Geometry: final body of the model. Coordinates: model frame, mm. A direction names the side the tool comes from. Round coordinates to 2 decimals unless told otherwise and drop trailing zeros. Loops run counter-clockwise (first coordinate to the right, second up) from the corner with the lowest first, then second, coordinate; pieces in that order, holes last. Notation, with made-up numbers: (-3, -24.5) - (3, -24.5) arc R32 cw to (3, 13.5) - close; hole circle Ø2 at (78.25, -4.75). An arc over 180 degrees is marked (long way). Answer as a JSON object with one key per item and string values. Group by question number.
Item 1: Line query: line 1 (Y direction, x = -15, z = -4.5); line 2 (X direction, y = 0.5, z = 7.75); line 3 (Y direction, x = -96, z = 1). Output: solid intervals per line, ascending.
Item 2: First-contact query: pin 1 (10 mm diameter, centred on x = -30, y = -24, fed in from -Z); pin 2 (8 mm diameter, centred on x = -88, y = 7.5, fed in from +Z); pin 3 (5 mm diameter, centred on x = -97, y = 13.5, fed in from +Z); pin 4 (3 mm diameter, centred on y = 6.5, z = -5.5, fed in from +X). Flat tips, straight axial feed; report the tip coordinate or a pass-through.
Item 3: Reachability of faces 1 (the face through (-9, -1, -0.042)), 2 (the face through (-102, 0, 5)), 3 (the face through (-82, 19, -4)), 4 (the face through (-3, 11, 6.958)) from +Z, -Z, +X, -X, +Y, -Y: full face, straight path, thin tool, end or side. Return the list, or none.
Item 4: Draft query along X for faces 5 (the face through (-102, 20, 5)), 6 (the face through (-82, -21, -4)), 7 (the face through (-2.292, 10.2, 7.4)), 8 (the face through (-72.292, -1, -4)). Return one class per face: released by +X, released by -X, zero draft, split by the parting line, or undercut.
Item 5: Section B-B (x = -33.5). Return the cut outline in (y, z).
Item 6: Section A-A (y = -22.5). Return the cut outline in (x, z).
```python
from build123d import *

# Parameters (mm, degrees)
BOSS_EXTRUDE1_DEPTH = 20
FILLET1_R           = 1
SKETCH2_R           = 9
CUT_EXTRUDE1_DEPTH  = 20
BOSS_EXTRUDE2_START = 2
BOSS_EXTRUDE2_DEPTH = 2
SKETCH4_W           = 20
SKETCH4_H           = 20
BOSS_EXTRUDE3_DEPTH = 2
FILLET2_R           = 1
SKETCH5_W           = 12.5
SKETCH5_H           = 2
CUT_EXTRUDE2_DEPTH  = 24
BOSS_EXTRUDE4_DEPTH = 80
FILLET3_R           = 1
SKETCH8_R           = 7.11392485
SKETCH8_W           = 20
SKETCH8_H           = 40
CUT_EXTRUDE3_DEPTH  = 2
SKETCH9_W           = 20
SKETCH9_H           = 2
BOSS_EXTRUDE5_DEPTH = 16
FILLET4_R           = 1
SKETCH10_R          = 2.5
CUT_EXTRUDE4_DEPTH  = 20


with BuildPart() as part:
    # Sketch1 → Boss-Extrude1 (new body)
    with BuildSketch(Plane(origin=(0, 0, 0), x_dir=(1, 0, 0), z_dir=(0, 1, 0))):
        Polygon((-2.291666667, 11.041666667), (-22.291666667, 11.041666667), (-22.291666667, -8.958333333), (-2.291666667, -8.958333333), (-2.291666667, -6.958333333), (-20.291666667, -6.958333333), (-20.291666667, 9.041666667), (-2.291666667, 9.041666667), align=None)
    extrude(amount=BOSS_EXTRUDE1_DEPTH)

    # Fillet1
    fillet1_edges = [part.edges().sort_by_distance(p)[0] for p in [
        (-22.291666667, 10, 8.958333333),
        (-22.291666667, 10, -11.041666667),
    ]]
    fillet(fillet1_edges, radius=FILLET1_R)

    # Sketch2 → Cut-Extrude1 (cut)
    with BuildSketch(Plane.XY.offset(8.958333333)):
        with Locations(Location((-12.291666667, 10, 0), (0, 0, 180))):
            Circle(SKETCH2_R)
    extrude(amount=-CUT_EXTRUDE1_DEPTH, mode=Mode.SUBTRACT)

    # Sketch3 → Boss-Extrude2 (add)
    with BuildSketch(Plane(origin=(0, 20, 0), x_dir=(1, 0, 0), z_dir=(0, 1, 0)).offset(BOSS_EXTRUDE2_START)):
        Polygon((-2.291666667, 2.377848536), (-2.291666667, 9.041666667), (-20.291666667, 9.041666667), (-20.291666667, -6.958333333), (-2.291666667, -6.958333333), (-2.291666667, 0.377848536), align=None)
        with BuildLine():
            Line((-2.291666667, 9.041666667), (-2.291666667, 11.041666667))
            Line((-2.291666667, 11.041666667), (-21.291666667, 11.041666667))
            ThreePointArc((-21.291666667, 11.041666667), (-21.998773448, 10.748773448), (-22.291666667, 10.041666667))
            Line((-22.291666667, 10.041666667), (-22.291666667, -7.958333333))
            ThreePointArc((-22.291666667, -7.958333333), (-21.998773448, -8.665440115), (-21.291666667, -8.958333333))
            Line((-21.291666667, -8.958333333), (-2.291666667, -8.958333333))
            Line((-2.291666667, -8.958333333), (-2.291666667, -6.958333333))
            Line((-2.291666667, -6.958333333), (-20.291666667, -6.958333333))
            Line((-20.291666667, -6.958333333), (-20.291666667, 9.041666667))
            Line((-20.291666667, 9.041666667), (-2.291666667, 9.041666667))
        make_face()
    extrude(amount=-BOSS_EXTRUDE2_DEPTH)

    # Sketch4 → Boss-Extrude3 (add)
    with BuildSketch(Plane.XZ):
        with Locations((-12.291666667, -1.041666667)):
            Rectangle(SKETCH4_W, SKETCH4_H)
    extrude(amount=BOSS_EXTRUDE3_DEPTH)

    # Fillet2
    fillet2_edges = [part.edges().sort_by_distance(p)[0] for p in [
        (-22.291666667, -1, -11.041666667),
        (-22.291666667, -1, 8.958333333),
    ]]
    fillet(fillet2_edges, radius=FILLET2_R - 0.0001)  # a hair under: the kernel refuses the full size

    # Sketch5 → Cut-Extrude2 (cut)
    with BuildSketch(Plane(origin=(0, 22, 0), x_dir=(1, 0, 0), z_dir=(0, 1, 0))):
        with Locations((-8.541666667, 1.041666667)):
            Rectangle(SKETCH5_W, SKETCH5_H)
    extrude(amount=-CUT_EXTRUDE2_DEPTH, mode=Mode.SUBTRACT)

    # Sketch6 → Boss-Extrude4 (add)
    with BuildSketch(Plane.ZY.offset(22.291666667)):
        Polygon((-2.491666667, -37), (-4.491666667, -37), (-4.491666667, -2), (-4.491666667, 22), (-2.491666667, 22), (-2.491666667, -2), align=None)
    extrude(amount=BOSS_EXTRUDE4_DEPTH)

    # Fillet3
    fillet3_edges = [part.edges().sort_by_distance(p)[0] for p in [
        (-22.291666667, -37, -3.491666667),
        (-102.291666667, 22, -3.491666667),
        (-102.291666667, -37, -3.491666667),
    ]]
    fillet(fillet3_edges, radius=FILLET3_R)

    # Sketch8 → Cut-Extrude3 (cut)
    with BuildSketch(Plane(origin=(0, 0, -4.491666667), x_dir=(-1, 0, 0), z_dir=(0, 0, -1))):
        with Locations((12.291666667, 10)):
            Circle(SKETCH8_R)
        with Locations((82.291666667, -1)):
            Rectangle(SKETCH8_W, SKETCH8_H)
    extrude(amount=-CUT_EXTRUDE3_DEPTH, mode=Mode.SUBTRACT)

    # Sketch9 → Boss-Extrude5 (add)
    with BuildSketch(Plane.XY.offset(-2.491666667)):
        Polygon((-92.823958121, 20), (-112.291666667, 20), (-112.291666667, 18), (-92.291666667, 18), (-92.291666667, 20), align=None)
        with Locations((-102.291666667, 1)):
            Rectangle(SKETCH9_W, SKETCH9_H)
    extrude(amount=BOSS_EXTRUDE5_DEPTH)

    # Fillet4
    fillet4_edges = [part.edges().sort_by_distance(p)[0] for p in [
        (-112.291666667, 19, -2.491666667),
        (-112.291666667, 19, 13.508333333),
        (-92.291666667, 19, 13.508333333),
        (-112.291666667, 1, -2.491666667),
        (-92.291666667, 1, 13.508333333),
        (-112.291666667, 1, 13.508333333),
    ]]
    fillet(fillet4_edges, radius=FILLET4_R)

    # Sketch10 → Cut-Extrude4 (cut)
    with BuildSketch(Plane(origin=(0, 20, 0), x_dir=(1, 0, 0), z_dir=(0, 1, 0))):
        with Locations(Location((-97.291666667, -5.508333333, 0), (0, 0, 180))):
            Circle(SKETCH10_R)
        with Locations(Location((-107.291666667, -5.508333333, 0), (0, 0, 180))):
            Circle(SKETCH10_R)
    extrude(amount=-CUT_EXTRUDE4_DEPTH, mode=Mode.SUBTRACT)


solid = part.part
```
Values:
{
 "1": {"line 1": "y = -2 to 0, 20 to 22", "line 2": "x = -112.29 to -108.4, -106.18 to -98.4, -96.18 to -92.29, -22.29 to -2.29", "line 3": "y = 0 to 2, 18 to 20"},
 "2": {"pin 1": "stops at z = -4.49", "pin 2": "passes through", "pin 3": "stops at z = -2.49", "pin 4": "stops at x = -20.29"},
 "3": {"face 1": "+X, +Y, -Y", "face 2": "+Z, -X, -Y", "face 3": "+Z, -Z", "face 4": "+X"},
 "4": {"face 5": "zero draft", "face 6": "undercut", "face 7": "released by +X", "face 8": "undercut"},
 "5": {"outline": "(-37, -4.49) - (22, -4.49) - (22, -2.49) - (-37, -2.49) - close"},
 "6": {"outline": "(-102.29, -4.49) - (-22.29, -4.49) - (-22.29, -2.49) - (-102.29, -2.49) - close"}
}
